from build123d import *

# Parameters (mm, degrees)
F1_DEPTH = 75
F3_DEPTH = 24.7
F4_DEPTH = 15.24
F5_DEPTH = 75


with BuildPart() as f1:
    # F0 (on Top) → F1 (new body)
    with BuildSketch(Plane.XY):
        Polygon((-126.0027056111, 215.9243343829), (-249.9973116764, -1.1593768134), (-123.9946060653, -217.0837111962), (126.0027056111, -215.9243343829), (249.9973116764, 1.1593768134), (123.9946060653, 217.0837111962), align=None)
    extrude(amount=F1_DEPTH)

    # F2 (on face) → F3 (cut)
    with BuildSketch(Plane.XY.offset(75)):
        Polygon((-105.9065815033, 175.3874490276), (-204.8432771145, -4.024065496), (-98.9366956112, -179.4115145236), (105.9065815033, -175.3874490276), (204.8432771145, 4.024065496), (98.9366956112, 179.4115145236), align=None)
    extrude(amount=-F3_DEPTH, mode=Mode.SUBTRACT)

    # F4 (cut): a face of the model
    f4_faces = [f1.faces().sort_by_distance(p)[0] for p in [
        (0, 0, 50.3),
    ]]
    extrude(f4_faces, amount=-F4_DEPTH, mode=Mode.SUBTRACT)

    # F5 (cut): a face of the model
    f5_faces = [f1.faces().sort_by_distance(p)[0] for p in [
        (0, 0, 35.06),
    ]]
    extrude(f5_faces, amount=-F5_DEPTH, mode=Mode.SUBTRACT)


solid = f1.part
Work out the finished part from the listing and answer in its coordinate system (mm). A direction names the side the tool comes from. Round coordinates to 2 decimals unless told otherwise and drop trailing zeros. Order: outer loops, then holes, each group sorted by start corner. A loop starts at its lowest first (then second) coordinate and runs counter-clockwise, first axis right, second up. Notation, with made-up numbers: M 1.25,81 L 32.25,81 A26 ccw 32.25,108 Z; hole C -20,31 d6. An arc over 180 degrees is marked long. One line per item, written item: value.
Q1. For faces 1 (the face through (-152.63, -90.49, 38.02)), 2 (the face through (-187.132, 108.902, 36.975)), determine the directions among +Z, -Z, +X, -X, +Y, -Y from which every point of the face is accessible in a straight line to the end or side of a thin tool.
Derived:
face 1: +Z, -Z
face 2: +Z, -Z, -X, +Y
Q2. Find section C-C on y = 169. Write down the section's boundary in (x, z).
Derived:
outline: M -152.81,0 L -109.43,0 L -109.43,75 L -152.81,75 Z; M 105.22,0 L 152.05,0 L 152.05,75 L 105.22,75 Z
Q3. Find section B-B on x = -116. Write down the section's boundary in (y, z), then the cut area to 3 significant figures.
Derived:
outline: M -217.05,0 L -151.15,0 L -151.15,75 L -217.05,75 Z; M 157.08,0 L 215.97,0 L 215.97,75 L 157.08,75 Z
area: 9,360 mm²
Q4. Find section A-A on z = 54.5. Write down the section's boundary in (x, y), then the cut area to 3 significant figures.
Derived:
outline: M -250,-1.16 L -123.99,-217.08 L 126,-215.92 L 250,1.16 L 123.99,217.08 L -126,215.92 Z; hole M -204.84,-4.02 L -98.94,-179.41 L 105.91,-175.39 L 204.84,4.02 L 98.94,179.41 L -105.91,175.39 Z
area: 53,300 mm²
Q5. Find section D-D on y = -186.5. Write down the section's boundary in (x, z), then the cut area to 3 significant figures.
Derived:
outline: M -141.84,0 L 142.81,0 L 142.81,75 L -141.84,75 Z
area: 21,300 mm²
Q6. Straight lines are drawn through the part: line 1 (X direction, y = 105.5, z = 18); line 2 (Y direction, x = -4.5, z = 69); line 3 (Y direction, x = -155.5, z = 55). For each, find the intervals that lie inside material, in ascending order.
Derived:
line 1: -189.08 to -144.45, 143.57 to 189.11
line 2: -216.53 to -177.56, 177.38 to 216.49
line 3: -163.09 to -85.74, 85.45 to 164.28
Q7. Flat-ended cylindrical pins translate along their axes: pin 1 (3 mm diameter, centred on x = 24, z = 49.5, fed in from +Y); pin 2 (4 mm diameter, centred on y = 104.5, z = 26, fed in from +X); pin 3 (2 mm diameter, centred on y = -58, z = 65.5, fed in from -X). Find the tip coordinate at first contact, or state that the pin passes through.
Derived:
pin 1: y = 216.63
pin 2: x = 190.86
pin 3: x = -217.41
Q8. Determine the mould class of faces 3 (the face through (-187.88, -107.61, 36.98)), 4 (the face through (154.68, -86.94, 38.02)), 5 (the face through (-20, 178, 75)) for opening direction Y: released by +Y, released by -Y, zero draft, split by the parting line, or undercut.
Derived:
face 3: released by -Y
face 4: undercut
face 5: zero draft
